```python
from build123d import *

# Parameters (mm, degrees)
SKETCH_3_R          = 75
EXTRUDE_1_DEPTH     = 25
SKETCH_4_R          = 25
EXTRUDE_3_DEPTH     = 5
EXTRUDE_START       = 5
SKETCH_6_R          = 25
EXTRUDE_4_DEPTH     = 5
CUT_EXTRUDE_3_DEPTH = 40


with BuildPart() as part:
    # 草图3 → 凸台-拉伸1 (new body)
    with BuildSketch(Plane(origin=(0, 0, 0), x_dir=(0, 0, -1), z_dir=(1, 0, 0))):
        Circle(SKETCH_3_R)
    extrude(amount=EXTRUDE_1_DEPTH)

    # 草图4 → 凸台-拉伸3 (add)
    with BuildSketch(Plane(origin=(25, 0, 0), x_dir=(0, 0, -1), z_dir=(1, 0, 0))):
        Circle(SKETCH_4_R)
    extrude(amount=EXTRUDE_3_DEPTH)

    # 草图6 → 凸台-拉伸4 (add)
    with BuildSketch(Plane.ZY.offset(EXTRUDE_START)):
        with Locations(Location((0, 0, 0), (0, 0, 180))):
            Circle(SKETCH_6_R)
    extrude(amount=-EXTRUDE_4_DEPTH)

    # 草图7 → 切除-拉伸3 (cut)
    with BuildSketch(Plane(origin=(30, 0, 0), x_dir=(0, 0, -1), z_dir=(1, 0, 0))):
        Polygon((7.366989435, 0), (3.683494717, 6.38), (-3.683494717, 6.38), (-7.366989435, 0), (-3.683494717, -6.38), (3.683494717, -6.38), align=None)
    extrude(amount=-CUT_EXTRUDE_3_DEPTH, mode=Mode.SUBTRACT)


solid = part.part
```
Design review of the part built by this model. Coordinates are the model's own, in mm. A direction names the side the tool comes from. Give positions to 0.01 mm unless a question says otherwise; leave off trailing zeros. Loops run counter-clockwise (first coordinate to the right, second up) from the corner with the lowest first, then second, coordinate; pieces in that order, holes last. Notation, with made-up numbers: M 86.5,38.5 L 108.5,38.5 A17 cw 108.5,57.5 Z; hole C -24,-38.75 d9. An arc over 180 degrees is marked long. Return JSON: item names as keys, results as strings. Group by question number.
Item 1: For probe 1 along X at (y, z) = (-38, 22.5); probe 2 along Y at (x, z) = (17, 0); probe 3 along Z at (x, y) = (27, -4), list the stretches that pass through material, from the lowest coordinate up.
Item 2: We need section D-D (z = 21). Give the boundary of the cut face in (x, y), and give its area (3 significant figures).
Item 3: We need section A-A (x = 16.5). Give the boundary of the cut face in (y, z).
Item 4: We need section B-B (z = 0). Give the boundary of the cut face in (x, y), and give its area (3 significant figures).
Item 5: Tool access review of faces 1 (the cylindrical face through (27.465, 7.509, -23.846)), 2 (the flat face through (30, -5, -5)), 3 (the flat face through (12.74, -3.15, 5.55)), 4 (the flat face through (0, 18, 18)): name each direction out of +Z, -Z, +X, -X, +Y, -Y from which nothing blocks a thin tool from reaching the whole face with its end or side.
Item 6: We need section C-C (y = -13.5). Give the boundary of the cut face in (x, z) (3 decimals).
Item 7: Insertion check: pin 1 Ø5 at (x, y) = (1, -36) entering from -Z; pin 2 Ø2 at (y, z) = (-36.5, 41) entering from -X; pin 3 Ø5 at (x, y) = (21.5, 44.5) entering from -Z. Each pin has a flat end and moves straight along its axis. Give the tip position at first contact, or say it passes through.
Item 8: Mouldability with a two-part tool opening along Y and no side actions: class faces 5 (the flat face through (13, -6.38, 0)), 6 (the cylindrical face through (-2.535, -7.509, -23.846)), 7 (the flat face through (25, 18, 18)) as released by +Y, released by -Y, zero draft, split by the parting line, or undercut.
Output:
{
 "1": {"probe 1": "x = 0 to 25", "probe 2": "y = -75 to -6.38, 6.38 to 75", "probe 3": "z = -24.68 to -5.06, 5.06 to 24.68"},
 "2": {"outline": "M -5,-13.56 L 0,-13.56 L 0,-72 L 25,-72 L 25,-13.56 L 30,-13.56 L 30,13.56 L 25,13.56 L 25,72 L 0,72 L 0,13.56 L -5,13.56 Z", "area": "3,870 mm^2"},
 "3": {"outline": "C 0,0 d150; hole M -6.38,-3.68 L 0,-7.37 L 6.38,-3.68 L 6.38,3.68 L 0,7.37 L -6.38,3.68 Z"},
 "4": {"outline": "M -5,-25 L 0,-25 L 0,-75 L 25,-75 L 25,-25 L 30,-25 L 30,-6.38 L -5,-6.38 Z; M -5,6.38 L 30,6.38 L 30,25 L 25,25 L 25,75 L 0,75 L 0,25 L -5,25 Z", "area": "3,800 mm^2"},
 "5": {"face 1": "+X", "face 2": "+Z, -Z, +X, +Y, -Y", "face 3": "+X, -X", "face 4": "-X"},
 "6": {"outline": "M -5,-21.042 L 0,-21.042 L 0,-73.775 L 25,-73.775 L 25,-21.042 L 30,-21.042 L 30,21.042 L 25,21.042 L 25,73.775 L 0,73.775 L 0,21.042 L -5,21.042 Z"},
 "7": {"pin 1": "stops at z = -67.1", "pin 2": "stops at x = 0", "pin 3": "stops at z = -62.14"},
 "8": {"face 5": "undercut", "face 6": "split by the parting line", "face 7": "zero draft"}
}
